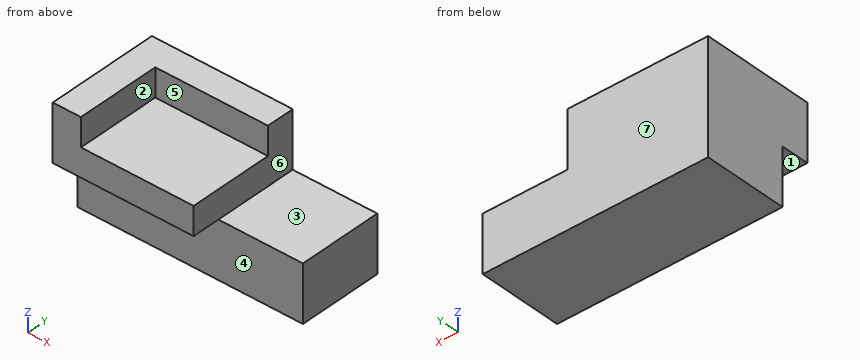
from build123d import *

# Parameters (mm, degrees)
F0_W     = 203.2
F0_H     = 76.2
F1_DEPTH = 50.8
F2_W     = 127
F2_H     = 76.2
F2_H_2   = 25.4
F3_DEPTH = 50.8
F4_W     = 101.6
F4_H     = 76.2
F5_DEPTH = 25.4
F6_ANGLE = 90


with BuildPart() as f1:
    # F0 (on Front) → F1 (new body)
    with BuildSketch(Plane.XZ):
        with Locations((-101.6, 38.1)):
            Rectangle(F0_W, F0_H)
    extrude(amount=F1_DEPTH)

    # F2 (on face) → F3 (join)
    with BuildSketch(Plane.XZ.offset(50.8)):
        with Locations((-139.7, 38.1)):
            Rectangle(F2_W, F2_H)
        with Locations((-139.7, -12.7)):
            Rectangle(F2_W, F2_H_2)
    extrude(amount=F3_DEPTH)

    # F4 (on face) → F5 (cut)
    with BuildSketch(Plane.XZ.offset(101.6)):
        with Locations((-127, 12.7)):
            Rectangle(F4_W, F4_H)
    extrude(amount=-F5_DEPTH, mode=Mode.SUBTRACT)


with BuildPart() as f1_1:
    # F6: moved
    add(f1.part.rotate(Axis((-101.6, 0, 0), (-1, 0, 0)), F6_ANGLE))


solid = f1_1.part
Could you check a few things on this model? Use its own coordinates, in mm. Face numbers are marked on the shaded views. A direction names the side the tool comes from. Give positions to 0.01 mm unless a question says otherwise; leave off trailing zeros. Write each loop counter-clockwise with the first axis right and the second up, starting at its lowest first coordinate (ties: lowest second). Pieces come first, ordered by that corner, then holes. Notation, with made-up numbers: (16.5, 28) -> (49.5, 28) arc R19 ccw to (49.5, 37) -> close; hole circle Ø1 at (28, 1.5). An arc over 180 degrees is marked (long way). Answer as a JSON object with one key per item and string values.
Q1. Suppose I cut it at D-D on y = -9.5. Write out the boundary of the cut face in (x, z).
Taken from the geometry:
{"outline": "(-203.2, 50.8) -> (-76.2, 50.8) -> (-76.2, 76.2) -> (-177.8, 76.2) -> (-177.8, 101.6) -> (-203.2, 101.6) -> close"}
Q2. Suppose I cut it at B-B on x = -126. Write out the boundary of the cut face in (y, z), then the cut area to 3 significant figures.
Taken from the geometry:
{"outline": "(-25.4, 50.8) -> (0, 50.8) -> (0, 0) -> (76.2, 0) -> (76.2, 101.6) -> (50.8, 101.6) -> (50.8, 76.2) -> (-25.4, 76.2) -> close", "area": "7,100 mm²"}
Q3. Which directions (+Z, -Z, +X, -X, +Y, -Y) give clear straight access to the entire face, cutting with the end or side of a thin tool? Please do the marked faces 4, 5, 6 and 7.
Taken from the geometry:
{"face 4": "-Z, +X, -X, -Y", "face 5": "+Z, +X, -Y", "face 6": "+Z, +X, +Y, -Y", "face 7": "+Z, -Z, +X, -X, +Y"}
Q4. Please list where these lines run through material, in increasing order: L1, parallel to X at y = -20, z = 59; L2, parallel to Z at x = -160.5, y = -15; L3, parallel to X at y = 32, z = 95.
Taken from the geometry:
{"L1": "x = -203.2 to -76.2", "L2": "z = 50.8 to 76.2", "L3": "x = -203.2 to -177.8"}
Q5. Suppose I cut it at C-C on z = 56.5. Write out the boundary of the cut face in (x, y).
Taken from the geometry:
{"outline": "(-203.2, -25.4) -> (-76.2, -25.4) -> (-76.2, 76.2) -> (-203.2, 76.2) -> close"}
Q6. We'd pull the mould along Z, two halves only. Please class the marked faces 1, 2 and 3: released by +Z, released by -Z, zero draft, split by the parting line, or undercut.
Taken from the geometry:
{"face 1": "released by -Z", "face 2": "zero draft", "face 3": "released by +Z"}
Q7. Will these pins go through, and if not, where does the flat tip stop? pin 1 Ø12.5 at (y, z) = (-6.5, 87) entering from +X; pin 2 Ø8 at (x, z) = (-91.5, 42) entering from -Y; pin 3 Ø12.5 at (x, y) = (-169, -15.5) entering from -Z; pin 4 Ø8 at (y, z) = (-5, 16.5) entering from +X.
Taken from the geometry:
{"pin 1": "stops at x = -177.8", "pin 2": "stops at y = 0", "pin 3": "stops at z = 50.8", "pin 4": "passes through"}
Q8. Suppose I cut it at A-A on y = 26.5. Write out the boundary of the cut face in (x, z), then the cut area to 3 significant figures.
Taken from the geometry:
{"outline": "(-203.2, 0) -> (0, 0) -> (0, 50.8) -> (-76.2, 50.8) -> (-76.2, 76.2) -> (-177.8, 76.2) -> (-177.8, 101.6) -> (-203.2, 101.6) -> close", "area": "14,200 mm²"}
